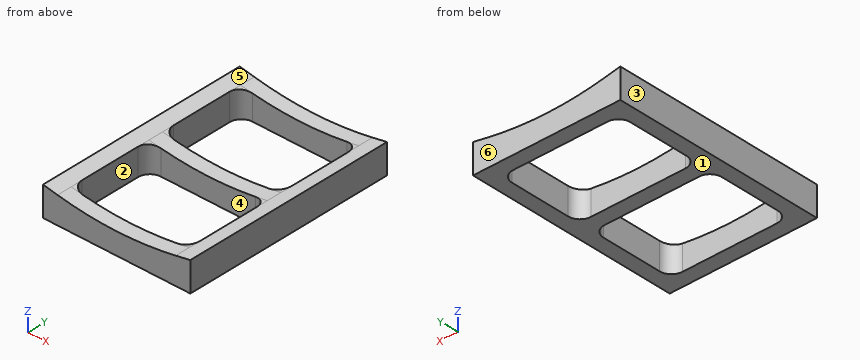
from build123d import *

# Parameters (mm, degrees)
F1_DEPTH     = 45.72
F2_DEPTH     = 39.37
F3_DEPTH     = 3.175
F4_T4_DEPTH  = 24.2661839103
F4_S5_R      = 142.2541111111
F4_T6_DEPTH  = 14
F4_T10_DEPTH = 24.2661839103
F4_S11_R     = 142.2541111111
F4_T12_DEPTH = 14
F4_T16_DEPTH = 24.2661839103
F4_S17_R     = 142.2541111111
F4_T18_DEPTH = 14
F4_T22_DEPTH = 24.2661839103
F4_S23_R     = 142.2541111111
F4_T24_DEPTH = 14
F4_T28_DEPTH = 24.2661839103
F4_S29_R     = 142.2541111111
F4_T30_DEPTH = 14
F4_T34_DEPTH = 24.2661839103
F4_S35_R     = 142.2541111111
F4_T36_DEPTH = 14
F4_T40_DEPTH = 24.2661839103
F4_S41_R     = 142.2541111111
F4_T42_DEPTH = 14
F4_T46_DEPTH = 24.2661839103
F4_S47_R     = 142.2541111111
F4_T48_DEPTH = 14


# Not quite as in the source:
# - a fillet or chamfer that OpenCascade refuses, or shapes differently, is made with other operations: its cross-section is extruded or revolved along the edge and cut away or added


with BuildPart() as f1:
    # F0 (on Front) → F1 (new body, symmetric)
    with BuildSketch(Plane.XZ):
        with BuildLine():
            ThreePointArc((25.4, 11.5661839103), (12.7513312638, 9.8528365344), (0, 9.2801839103))
            ThreePointArc((0, 9.2801839103), (-12.7513312638, 9.8528365344), (-25.4, 11.5661839103))
            Line((-25.4, 11.5661839103), (-25.4, 0))
            Line((-25.4, 0), (25.4, 0))
            Line((25.4, 0), (25.4, 11.5661839103))
        make_face()
        Polygon((-25.4, 0), (-25.4, 11.5661839103), (-31.6479565519, 12.7), (-31.6479565519, 0), align=None)
        Polygon((31.6479565519, 12.7), (25.4, 11.5661839103), (25.4, 0), (31.6479565519, 0), align=None)
    extrude(amount=F1_DEPTH, both=True)

    # F0 (on Front) → F2 (cut, symmetric)
    with BuildSketch(Plane.XZ):
        with BuildLine():
            ThreePointArc((25.4, 11.5661839103), (12.7513312638, 9.8528365344), (0, 9.2801839103))
            ThreePointArc((0, 9.2801839103), (-12.7513312638, 9.8528365344), (-25.4, 11.5661839103))
            Line((-25.4, 11.5661839103), (-25.4, 0))
            Line((-25.4, 0), (25.4, 0))
            Line((25.4, 0), (25.4, 11.5661839103))
        make_face()
    extrude(amount=F2_DEPTH, both=True, mode=Mode.SUBTRACT)

    # F0 (on Front) → F3 (join, symmetric)
    with BuildSketch(Plane.XZ):
        with BuildLine():
            ThreePointArc((25.4, 11.5661839103), (12.7513312638, 9.8528365344), (0, 9.2801839103))
            ThreePointArc((0, 9.2801839103), (-12.7513312638, 9.8528365344), (-25.4, 11.5661839103))
            Line((-25.4, 11.5661839103), (-25.4, 0))
            Line((-25.4, 0), (25.4, 0))
            Line((25.4, 0), (25.4, 11.5661839103))
        make_face()
    extrude(amount=F3_DEPTH, both=True)

    # F4: fillet of radius 5.08 on 8 edges, made by hand


with BuildPart() as f4_tool2:
    # F4_s3 → F4_t4 (new body)
    with BuildSketch(Plane.XY.offset(24.2661839103)):
        with BuildLine():
            ThreePointArc((-20.32, 39.37), (-23.9121024484, 37.8821024484), (-25.4, 34.29))
            Line((-25.4, 34.29), (-25.4, 39.37))
            Line((-25.4, 39.37), (-20.32, 39.37))
        make_face()
    extrude(amount=-F4_T4_DEPTH)

    # F4_s5 → F4_t6 (cut, symmetric)
    with BuildSketch(Plane.XZ.offset(-36.8)):
        with Locations((0, 151.5342950214)):
            Circle(F4_S5_R)
    extrude(amount=F4_T6_DEPTH, both=True, mode=Mode.SUBTRACT)


with BuildPart() as f1_1:
    add(f1.part)

    # F4_t1: union F4_tool2
    add(f4_tool2.part)


with BuildPart() as f4_tool8:
    # F4_s9 → F4_t10 (new body)
    with BuildSketch(Plane.XY):
        with BuildLine():
            ThreePointArc((20.32, 39.37), (23.9121024484, 37.8821024484), (25.4, 34.29))
            Line((25.4, 34.29), (25.4, 39.37))
            Line((25.4, 39.37), (20.32, 39.37))
        make_face()
    extrude(amount=F4_T10_DEPTH)

    # F4_s11 → F4_t12 (cut, symmetric)
    with BuildSketch(Plane.XZ.offset(-36.8)):
        with Locations((0, 151.5342950214)):
            Circle(F4_S11_R)
    extrude(amount=F4_T12_DEPTH, both=True, mode=Mode.SUBTRACT)


with BuildPart() as f1_2:
    add(f1_1.part)

    # F4_t7: union F4_tool8
    add(f4_tool8.part)


with BuildPart() as f4_tool14:
    # F4_s15 → F4_t16 (new body)
    with BuildSketch(Plane.XY):
        with BuildLine():
            ThreePointArc((25.4, -8.255), (23.9121024484, -4.6628975516), (20.32, -3.175))
            Line((20.32, -3.175), (25.4, -3.175))
            Line((25.4, -3.175), (25.4, -8.255))
        make_face()
    extrude(amount=F4_T16_DEPTH)

    # F4_s17 → F4_t18 (cut, symmetric)
    with BuildSketch(Plane.XZ.offset(5.7)):
        with Locations((0, 151.5342950214)):
            Circle(F4_S17_R)
    extrude(amount=F4_T18_DEPTH, both=True, mode=Mode.SUBTRACT)


with BuildPart() as f1_3:
    add(f1_2.part)

    # F4_t13: union F4_tool14
    add(f4_tool14.part)


with BuildPart() as f4_tool20:
    # F4_s21 → F4_t22 (new body)
    with BuildSketch(Plane.XY.offset(24.2661839103)):
        with BuildLine():
            ThreePointArc((-25.4, -8.255), (-23.9121024484, -4.6628975516), (-20.32, -3.175))
            Line((-20.32, -3.175), (-25.4, -3.175))
            Line((-25.4, -3.175), (-25.4, -8.255))
        make_face()
    extrude(amount=-F4_T22_DEPTH)

    # F4_s23 → F4_t24 (cut, symmetric)
    with BuildSketch(Plane.XZ.offset(5.7)):
        with Locations((0, 151.5342950214)):
            Circle(F4_S23_R)
    extrude(amount=F4_T24_DEPTH, both=True, mode=Mode.SUBTRACT)


with BuildPart() as f1_4:
    add(f1_3.part)

    # F4_t19: union F4_tool20
    add(f4_tool20.part)


with BuildPart() as f4_tool26:
    # F4_s27 → F4_t28 (new body)
    with BuildSketch(Plane.XY):
        with BuildLine():
            ThreePointArc((25.4, 8.255), (23.9121024484, 4.6628975516), (20.32, 3.175))
            Line((20.32, 3.175), (25.4, 3.175))
            Line((25.4, 3.175), (25.4, 8.255))
        make_face()
    extrude(amount=F4_T28_DEPTH)

    # F4_s29 → F4_t30 (cut, symmetric)
    with BuildSketch(Plane.XZ.offset(-5.7)):
        with Locations((0, 151.5342950214)):
            Circle(F4_S29_R)
    extrude(amount=F4_T30_DEPTH, both=True, mode=Mode.SUBTRACT)


with BuildPart() as f1_5:
    add(f1_4.part)

    # F4_t25: union F4_tool26
    add(f4_tool26.part)


with BuildPart() as f4_tool32:
    # F4_s33 → F4_t34 (new body)
    with BuildSketch(Plane.XY):
        with BuildLine():
            ThreePointArc((25.4, -34.29), (23.9121024484, -37.8821024484), (20.32, -39.37))
            Line((20.32, -39.37), (25.4, -39.37))
            Line((25.4, -39.37), (25.4, -34.29))
        make_face()
    extrude(amount=F4_T34_DEPTH)

    # F4_s35 → F4_t36 (cut, symmetric)
    with BuildSketch(Plane.XZ.offset(36.8)):
        with Locations((0, 151.5342950214)):
            Circle(F4_S35_R)
    extrude(amount=F4_T36_DEPTH, both=True, mode=Mode.SUBTRACT)


with BuildPart() as f1_6:
    add(f1_5.part)

    # F4_t31: union F4_tool32
    add(f4_tool32.part)


with BuildPart() as f4_tool38:
    # F4_s39 → F4_t40 (new body)
    with BuildSketch(Plane.XY.offset(24.2661839103)):
        with BuildLine():
            ThreePointArc((-25.4, -34.29), (-23.9121024484, -37.8821024484), (-20.32, -39.37))
            Line((-20.32, -39.37), (-25.4, -39.37))
            Line((-25.4, -39.37), (-25.4, -34.29))
        make_face()
    extrude(amount=-F4_T40_DEPTH)

    # F4_s41 → F4_t42 (cut, symmetric)
    with BuildSketch(Plane.XZ.offset(36.8)):
        with Locations((0, 151.5342950214)):
            Circle(F4_S41_R)
    extrude(amount=F4_T42_DEPTH, both=True, mode=Mode.SUBTRACT)


with BuildPart() as f1_7:
    add(f1_6.part)

    # F4_t37: union F4_tool38
    add(f4_tool38.part)


with BuildPart() as f4_tool44:
    # F4_s45 → F4_t46 (new body)
    with BuildSketch(Plane.XY.offset(24.2661839103)):
        with BuildLine():
            ThreePointArc((-25.4, 8.255), (-23.9121024484, 4.6628975516), (-20.32, 3.175))
            Line((-20.32, 3.175), (-25.4, 3.175))
            Line((-25.4, 3.175), (-25.4, 8.255))
        make_face()
    extrude(amount=-F4_T46_DEPTH)

    # F4_s47 → F4_t48 (cut, symmetric)
    with BuildSketch(Plane.XZ.offset(-5.7)):
        with Locations((0, 151.5342950214)):
            Circle(F4_S47_R)
    extrude(amount=F4_T48_DEPTH, both=True, mode=Mode.SUBTRACT)


with BuildPart() as f1_8:
    add(f1_7.part)

    # F4_t43: union F4_tool44
    add(f4_tool44.part)


solid = f1_8.part
Read the model definition and answer for the solid it produces. Units are mm, in the model's axes. Face numbers are marked on the shaded views. A direction names the side the tool comes from. Coordinates: 2 decimals unless noted, no trailing zeros. Order: outer loops, then holes, each group sorted by start corner. A loop starts at its lowest first (then second) coordinate and runs counter-clockwise, first axis right, second up. Notation, with made-up numbers: M 15.25,-21 L 29.25,-21 A24 ccw 29.25,-11 Z; hole C 61.25,15 d10. An arc over 180 degrees is marked long. Put each result on its own line as item: value. Start each with the question number.
Item 1: Consider probe 1 along Y at (x, z) = (-10, 5.5) (3 decimals); probe 2 along X at (y, z) = (-10.5, 6.25); probe 3 along Y at (x, z) = (21.5, 10.25). Determine where each line is inside the solid, lowest interval first. Write a range as [from, to].
Item 2: For the marked faces 4, 5 and 6, determine the directions among +Z, -Z, +X, -X, +Y, -Y from which every point of the face is accessible in a straight line to the end or side of a thin tool.
Item 3: Section A-A, the plane y = -17 is taken. Determine the outline of the cut face in (x, z).
Item 4: Given pin 1 Ø4 at (x, y) = (13.5, -5) entering from +Z, flat-ended and moving along its own axis, determine where the tip first touches the part or whether it passes through.
Item 5: Section B-B, the plane x = -6 is taken. Determine the outline of the cut face in (y, z) (3 decimals), plus the area to 3 significant figures.
Item 6: Section D-D, the plane y = 0 is taken. Determine the outline of the cut face in (x, z), plus the area to 3 significant figures.
Item 7: Section C-C, the plane z = 5.25 is taken. Determine the outline of the cut face in (x, y) (3 decimals), plus the area to 3 significant figures.
Item 8: The mould has two halves that part along X. Classify the marked faces 1, 2 and 3: +X half, -X half, draft (parallel to the pull), parting line (faces both ways), or undercut.
Computed:
1. probe 1: y = [-45.72, -39.37], [-3.175, 3.175], [39.37, 45.72]
1. probe 2: x = [-31.65, -25.4], [25.4, 31.65]
1. probe 3: y = [-45.72, -39.23], [-3.31, 3.31], [39.23, 45.72]
2. face 4: +Z, -Z
2. face 5: +Z, +Y, -Y
2. face 6: +Z, -Z, +X, -X, +Y
3. outline: M -31.65,0 L -25.4,0 L -25.4,11.57 L -31.65,12.7 Z; M 25.4,0 L 31.65,0 L 31.65,12.7 L 25.4,11.57 Z
4. pin 1: stops at z = 10
5. outline: M -45.72,0 L -39.37,0 L -39.37,9.407 L -45.72,9.407 Z; M -3.175,0 L 3.175,0 L 3.175,9.407 L -3.175,9.407 Z; M 39.37,0 L 45.72,0 L 45.72,9.407 L 39.37,9.407 Z
5. area: 179 mm2
6. outline: M -31.65,0 L 31.65,0 L 31.65,12.7 L 25.4,11.57 A142.25 cw -25.4,11.57 L -31.65,12.7 Z
6. area: 662 mm2
7. outline: M -31.648,-45.72 L 31.648,-45.72 L 31.648,45.72 L -31.648,45.72 Z; hole M -25.4,-34.29 A5.08 ccw -20.32,-39.37 L 20.32,-39.37 A5.08 ccw 25.4,-34.29 L 25.4,-8.255 A5.08 ccw 20.32,-3.175 L -20.32,-3.175 A5.08 ccw -25.4,-8.255 Z; hole M -25.4,8.255 A5.08 ccw -20.32,3.175 L 20.32,3.175 A5.08 ccw 25.4,8.255 L 25.4,34.29 A5.08 ccw 20.32,39.37 L -20.32,39.37 A5.08 ccw -25.4,34.29 Z
7. area: 2,150 mm2
8. face 1: draft
8. face 2: undercut
8. face 3: -X half
